```python
from build123d import *

# Parameters (mm, degrees)
F1_ANGLE = 265


with BuildPart() as f1:
    # F0 (on Top) → F1 (revolve)
    with BuildSketch(Plane.XY):
        Polygon((25.4, 50.8), (0, 50.8), (0, 44.253774), (18.482406, 44.253774), (18.482406, -44.45), (25.4, -44.45), align=None)
        Polygon((25.4, -50.8), (25.4, -44.45), (18.482406, -44.45), (4.925116, -44.45), (4.925116, -50.8), align=None)
    revolve(axis=Axis((0, 25.4, 0), (0, 1, 0)), revolution_arc=F1_ANGLE)


solid = f1.part
```
Can you work these out from the model? Positions are in its coordinate system, mm. A direction names the side the tool comes from. Round coordinates to 2 decimals unless told otherwise and drop trailing zeros. Loops run counter-clockwise (first coordinate to the right, second up) from the corner with the lowest first, then second, coordinate; pieces in that order, holes last.
Item 1: Suppose I cut it at B-B, the plane z = -2. Write out the boundary of the cut face in (x, y), then the cut area to 3 significant figures.
Item 2: Suppose I cut it at D-D, the plane y = 41.5. Write out the boundary of the cut face in (x, z), then the cut area to 3 significant figures.
Item 3: Which directions (+Z, -Z, +X, -X, +Y, -Y) give clear straight access to the entire face, cutting with the end or side of a thin tool? Please do faces 5 (the cylindrical face through (-3.208, -47.669, -3.737)), 6 (the flat face through (-4, -44.45, -4)), 7 (the flat face through (-1.676, 4, 19.153)).
Item 4: Suppose I cut it at A-A, the plane x = -6.5. Write out the boundary of the cut face in (y, z), then the cut area to 3 significant figures.
Item 5: Suppose I cut it at C-C, the plane x = 13. Write out the boundary of the cut face in (y, z).
Item 6: If we mould it in two halves opening along Y, with no side actions, what happens to faces 1 (the flat face through (19, 4, 0)), 2 (the cylindrical face through (-12.039, -0.719, -14.024)), 3 (the flat face through (-6, 50.8, -6)), 4 (the flat face through (-5, -50.8, -6))? For each: +Y half, -Y half, draft (parallel to the pull), parting line (faces both ways), or undercut.
Item 7: Will these pins go through, and if not, where does the flat tip stop? pin 1 Ø3 at (y, z) = (-15.5, 11.5) entering from -X; pin 2 Ø8 at (x, y) = (-7, -14) entering from +Z; pin 3 Ø1.5 at (y, z) = (-34, -13) entering from -X.
Item 8: Please list where these lines run through material, in increasing order: L1, parallel to Y at x = -2.5, z = 8; L2, parallel to Z at x = 0, y = -46.75; L3, parallel to X at y = 44, z = -17.
Reported:
1. outline: (-25.32, -50.8) - (-4.5, -50.8) - (-4.5, -44.45) - (-18.37, -44.45) - (-18.37, 44.25) - (18.37, 44.25) - (18.37, -44.45) - (4.5, -44.45) - (4.5, -50.8) - (25.32, -50.8) - (25.32, 50.8) - (-25.32, 50.8) - close
1. area: 1,830 mm2
2. outline: (-2.21, 25.3) arc R25.4 ccw (long way) to (25.4, 0) - (18.48, 0) arc R18.48 cw (long way) to (-1.61, 18.41) - close
2. area: 702 mm2
3. face 5: -Y
3. face 6: none
3. face 7: +Z, +X, +Y, -Y
4. outline: (-50.8, -24.55) - (50.8, -24.55) - (50.8, 24.55) - (-50.8, 24.55) - close; hole (-44.45, -17.3) - (44.25, -17.3) - (44.25, 17.3) - (-44.45, 17.3) - close
4. area: 1,920 mm2
5. outline: (-50.8, -21.82) - (50.8, -21.82) - (50.8, 0) - (44.25, 0) - (44.25, -13.14) - (-44.45, -13.14) - (-44.45, 0) - (-50.8, 0) - close
6. face 1: draft
6. face 2: undercut
6. face 3: +Y half
6. face 4: -Y half
7. pin 1: stops at x = -23.35
7. pin 2: stops at z = 25.22
7. pin 3: stops at x = -22.25
8. L1: y = -50.8 to -44.45, 44.25 to 50.8
8. L2: z = -25.4 to -4.93
8. L3: x = -18.87 to -7.25, 7.25 to 18.87
